Can you work these out from the model? Positions are in its coordinate system, mm. A direction names the side the tool comes from. Round coordinates to 2 decimals unless told otherwise and drop trailing zeros. Write each loop counter-clockwise with the first axis right and the second up, starting at its lowest first coordinate (ties: lowest second). Pieces come first, ordered by that corner, then holes. Notation, with made-up numbers: M -15.75,57.25 L 12.25,57.25 A8 ccw 12.25,63.25 Z; hole C 23,-35.5 d3. An arc over 180 degrees is marked long. Answer in a Markdown table with one row per item. Add a question column.
(1) If I drill on probe 1 along Z at (x, y) = (11, 6.5); probe 2 along Z at (x, y) = (40, -25.5); probe 3 along Y at (x, z) = (16, 40.5), over which ranges is the centre line in solid material (lowest first)?
(2) Suppose I cut it at C-C, the plane x = 40. Write out the boundary of the cut face in (y, z), then the cut area to 3 significant figures.
(3) I'm going to push flat-ended pins straight in: pin 1 (24.5 mm diameter, centred on x = 28, y = -6, fed in from +Z); pin 2 (4 mm diameter, centred on x = 36.5, z = 12, fed in from +Y); pin 3 (3 mm diameter, centred on x = 19.5, y = 19, fed in from -Z). Where does each tip first touch, or does it pass through?
(4) For faces 1 (the face through (12.407, 29.843, -4.696)), 2 (the face through (24, -12.7, 32)), 3 (the face through (24, 12.7, 32)), 4 (the face through (1, -37, 0)), which set-ups out of +Z, -Z, +X, -X, +Y, -Y let a thin tool reach every point of the face, with its end or its side?
(5) Suppose I cut it at B-B, the plane y = -28.5. Write out the boundary of the cut face in (x, z) (3 decimals), then the cut area to 3 significant figures.
(6) Suppose I cut it at D-D, the plane z = 38.5. Write out the boundary of the cut face in (x, y), then the cut area to 3 significant figures.
(7) If we mould it in two halves opening along X, with no side actions, what happens to faces 5 (the face through (5.523, -38.046, -4.696)), 6 (the face through (0, -1, 4)), 7 (the face through (5.133, 0.178, 53.646)), 8 (the face through (1, 37, 0))? For each: released by +X, released by -X, zero draft, split by the parting line, or undercut.
(8) Suppose I cut it at A-A, the plane y = 4. Write out the boundary of the cut face in (x, z), then the cut area to 3 significant figures.
from build123d import *

# Parameters (mm, degrees)
F1_DEPTH = 38.1
F0_R     = 2.445033
F2_DEPTH = 12.7
F3_R     = 6.35
F4_DEPTH = 9.525


with BuildPart() as f1:
    # F0 (on Front) → F1 (new body, symmetric)
    with BuildSketch(Plane.XZ):
        Polygon((0, 7.562613), (0, 0), (48.733659, 0), (48.733659, 7.562613), (37.851159, 7.562613), (20.859193, 7.562613), align=None)
    extrude(amount=F1_DEPTH, both=True)

    # F0 (on Front) → F2 (join, symmetric)
    with BuildSketch(Plane.XZ):
        with BuildLine():
            ThreePointArc((3.904653, 47.668676), (20.394154, 31.002756), (20.859193, 7.562613))
            Line((20.859193, 7.562613), (37.851159, 7.562613))
            ThreePointArc((37.851159, 7.562613), (29.868225, 36.114692), (6.873098, 54.82759))
            ThreePointArc((6.873098, 54.82759), (1.871612, 52.706566), (3.904653, 47.668676))
        make_face()
        with Locations((5.451619, 51.222116)):
            Circle(F0_R, mode=Mode.SUBTRACT)
    extrude(amount=F2_DEPTH, both=True)

    # F3 (on face) → F4 (join)
    with BuildSketch(Plane(origin=(0, 0, 0), x_dir=(1, 0, 0), z_dir=(0, 0, -1))):
        with Locations((6.35, -31.75)):
            Circle(F3_R)
        with Locations((6.35, 31.75)):
            Circle(F3_R)
    extrude(amount=F4_DEPTH)


solid = f1.part
Calculated:
| question | item | result |
|---|---|---|
| 1 | probe 1 | 0 to 7.56, 43.4 to 52.98 |
| 1 | probe 2 | 0 to 7.56 |
| 1 | probe 3 | -12.7 to 12.7 |
| 2 | outline | M -38.1,0 L 38.1,0 L 38.1,7.56 L -38.1,7.56 Z |
| 2 | area | 576 mm² |
| 3 | pin 1 | z = 50.23 |
| 3 | pin 2 | y = 12.7 |
| 3 | pin 3 | z = 0 |
| 4 | face 1 | -Z |
| 4 | face 2 | +Z, +X, -X, -Y |
| 4 | face 3 | +Z, +X, -X, +Y |
| 4 | face 4 | -Z, -X, -Y |
| 5 | outline | M 0,0 L 0.895,0 L 0.895,-9.525 L 11.805,-9.525 L 11.805,0 L 48.734,0 L 48.734,7.563 L 0,7.563 Z |
| 5 | area | 472 mm² |
| 6 | outline | M 15.91,-12.7 L 28.2,-12.7 L 28.2,12.7 L 15.91,12.7 Z |
| 6 | area | 312 mm² |
| 7 | face 5 | split by the parting line |
| 7 | face 6 | released by -X |
| 7 | face 7 | undercut |
| 7 | face 8 | zero draft |
| 8 | outline | M 0,0 L 48.73,0 L 48.73,7.56 L 37.85,7.56 A48.97 ccw 6.87,54.83 A3.88 ccw 3.9,47.67 A31.59 cw 20.86,7.56 L 0,7.56 Z; hole C 5.45,51.22 d4.89 |
| 8 | area | 979 mm² |
